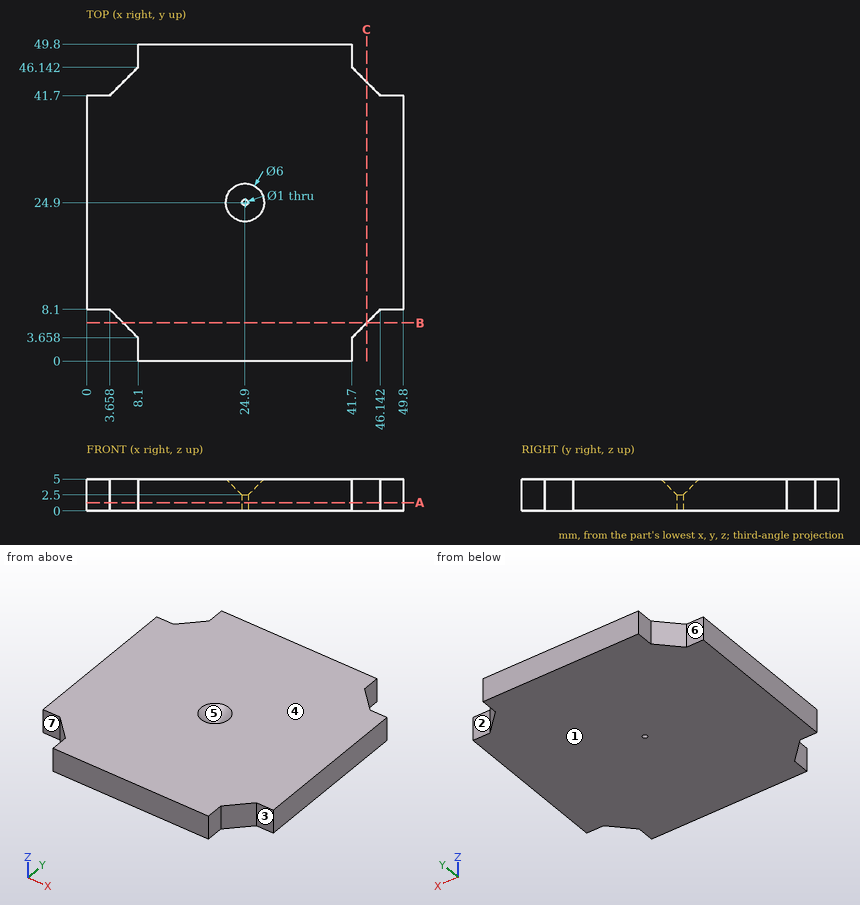
Can you work these out from the drawing? Everything is in mm from the part's minimum corner. A direction names the side the tool comes from. Give positions to 0.01 mm unless a question says otherwise; leave off trailing zeros. Write each loop counter-clockwise with the first axis right and the second up, starting at its lowest first coordinate (ties: lowest second). Pieces come first, ordered by that corner, then holes. Notation, with made-up numbers: (87.5, 47) -> (123.5, 47) arc R19 cw to (123.5, 69) -> close; hole circle Ø7 at (31, -21). An arc over 180 degrees is marked (long way). Write each question's results on one line, items separated by ' | '. Start each with the question number.
Q1. We'd pull the mould along Y, two halves only. Please class the marked faces 4, 5, 6 and 7: +Y half, -Y half, draft (parallel to the pull), parting line (faces both ways), or undercut.
Q2. Suppose I cut it at B-B, the plane y = 6. List the corners of the cut face in (x, z) for me, and give its area (3 significant figures).
Q3. Which directions (+Z, -Z, +X, -X, +Y, -Y) give clear straight access to the entire face, cutting with the end or side of a thin tool? Please do the marked faces 1, 2 and 3.
Q4. Suppose I cut it at C-C, the plane x = 44. List the corners of the cut face in (y, z) for me.
Q5. I need wall thicknesses on probe 1 along X at (y, z) = (24.9, 1.3); probe 2 along Y at (x, z) = (4.5, 0.4); probe 3 along X at (y, z) = (6, 1.3). Which ranges of each line are inside material? Lowest first, please.
Q6. Suppose I cut it at A-A, the plane z = 1.3. List the corners of the cut face in (x, y) for me.
Q7. I'm going to push flat-ended pins straight in: pin 1 Ø1.1 at (y, z) = (49, 3) entering from +X; pin 2 Ø1.8 at (x, z) = (2, 2.5) entering from -Y; pin 3 Ø1.8 at (y, z) = (47.5, 2.5) entering from -X; pin 4 Ø1 at (x, y) = (32.5, 18) entering from -Z. Where does each tip first touch, or does it pass through?
Outcome:
1) face 4: draft | face 5: undercut | face 6: +Y half | face 7: -Y half
2) outline: (5.76, 0) -> (44.04, 0) -> (44.04, 5) -> (5.76, 5) -> close | area: 191 mm2
3) face 1: -Z, +X, -X, +Y, -Y | face 2: +Z, -Z, +X, +Y | face 3: +Z, -Z, +X, -Y
4) outline: (5.96, 0) -> (43.84, 0) -> (43.84, 5) -> (5.96, 5) -> close
5) probe 1: 0 to 24.4, 25.4 to 49.8 | probe 2: 7.26 to 42.54 | probe 3: 5.76 to 44.04
6) outline: (0, 8.1) -> (3.66, 8.1) -> (8.1, 3.66) -> (8.1, 0) -> (41.7, 0) -> (41.7, 3.66) -> (46.14, 8.1) -> (49.8, 8.1) -> (49.8, 41.7) -> (46.14, 41.7) -> (41.7, 46.14) -> (41.7, 49.8) -> (8.1, 49.8) -> (8.1, 46.14) -> (3.66, 41.7) -> (0, 41.7) -> close; hole circle Ø1 at (24.9, 24.9)
7) pin 1: x = 41.7 | pin 2: y = 8.1 | pin 3: x = 8.1 | pin 4: z = 0
